from build123d import *

# Parameters (mm, degrees)
F1_DEPTH = 3
F2_DEPTH = 17
F3_R     = 5
F4_R     = 5
F5_R     = 2


with BuildPart() as f1:
    # F0 (on Top) → F1 (new body)
    with BuildSketch(Plane.XY):
        Polygon((-13.561376, 18.665632), (-57.446909, 18.665632), (-21.942767, -7.129637), (-35.504142, -48.867259), (0, -23.07199), (35.504142, -48.867259), (21.942767, -7.129637), (57.446909, 18.665632), (13.561376, 18.665632), (0, 60.403254), align=None)
        with BuildLine():
            Line((-37.903616, 13.665631), (-9.928662, 13.665631))
            Line((-9.928662, 13.665631), (-1.283926, 40.271394))
            ThreePointArc((-1.283926, 40.271394), (0, 41.204221), (1.283926, 40.271394))
            Line((1.283926, 40.271394), (9.928662, 13.665631))
            Line((9.928662, 13.665631), (37.903616, 13.665631))
            ThreePointArc((37.903616, 13.665631), (39.187542, 12.732804), (38.697126, 11.223459))
            Line((38.697126, 11.223459), (16.064913, -5.219807))
            Line((16.064913, -5.219807), (24.709649, -31.825569))
            ThreePointArc((24.709649, -31.825569), (24.219233, -33.334915), (22.632213, -33.334915))
            Line((22.632213, -33.334915), (0, -16.891649))
            Line((0, -16.891649), (-22.632213, -33.334915))
            ThreePointArc((-22.632213, -33.334915), (-24.219233, -33.334915), (-24.709649, -31.825569))
            Line((-24.709649, -31.825569), (-16.064913, -5.219807))
            Line((-16.064913, -5.219807), (-38.697126, 11.223459))
            ThreePointArc((-38.697126, 11.223459), (-39.187542, 12.732804), (-37.903616, 13.665631))
        make_face(mode=Mode.SUBTRACT)
        with BuildLine():
            Line((-1.283926, 40.271394), (-9.928662, 13.665631))
            Line((-9.928662, 13.665631), (-37.903616, 13.665631))
            ThreePointArc((-37.903616, 13.665631), (-39.187542, 12.732804), (-38.697126, 11.223459))
            Line((-38.697126, 11.223459), (-16.064913, -5.219807))
            Line((-16.064913, -5.219807), (-24.709649, -31.825569))
            ThreePointArc((-24.709649, -31.825569), (-24.219233, -33.334915), (-22.632213, -33.334915))
            Line((-22.632213, -33.334915), (0, -16.891649))
            Line((0, -16.891649), (22.632213, -33.334915))
            ThreePointArc((22.632213, -33.334915), (24.219233, -33.334915), (24.709649, -31.825569))
            Line((24.709649, -31.825569), (16.064913, -5.219807))
            Line((16.064913, -5.219807), (38.697126, 11.223459))
            ThreePointArc((38.697126, 11.223459), (39.187542, 12.732804), (37.903616, 13.665631))
            Line((37.903616, 13.665631), (9.928662, 13.665631))
            Line((9.928662, 13.665631), (1.283926, 40.271394))
            ThreePointArc((1.283926, 40.271394), (0, 41.204221), (-1.283926, 40.271394))
        make_face()
        with BuildLine():
            Line((-23.948804, -32.072782), (-15.124457, -4.914234))
            Line((-15.124457, -4.914234), (-38.226898, 11.870672))
            ThreePointArc((-38.226898, 11.870672), (-38.426697, 12.485591), (-37.903616, 12.865631))
            Line((-37.903616, 12.865631), (-9.347428, 12.865631))
            Line((-9.347428, 12.865631), (-0.523081, 40.02418))
            ThreePointArc((-0.523081, 40.02418), (0, 40.404221), (0.523081, 40.02418))
            Line((0.523081, 40.02418), (9.347428, 12.865631))
            Line((9.347428, 12.865631), (37.903616, 12.865631))
            ThreePointArc((37.903616, 12.865631), (38.426697, 12.485591), (38.226898, 11.870672))
            Line((38.226898, 11.870672), (15.124457, -4.914234))
            Line((15.124457, -4.914234), (23.948804, -32.072782))
            ThreePointArc((23.948804, -32.072782), (23.749005, -32.687701), (23.102441, -32.687701))
            Line((23.102441, -32.687701), (0, -15.902795))
            Line((0, -15.902795), (-23.102441, -32.687701))
            ThreePointArc((-23.102441, -32.687701), (-23.749005, -32.687701), (-23.948804, -32.072782))
        make_face(mode=Mode.SUBTRACT)
    extrude(amount=-F1_DEPTH)

    # F0 (on Top) → F2 (join)
    with BuildSketch(Plane.XY):
        with BuildLine():
            Line((-1.283926, 40.271394), (-9.928662, 13.665631))
            Line((-9.928662, 13.665631), (-37.903616, 13.665631))
            ThreePointArc((-37.903616, 13.665631), (-39.187542, 12.732804), (-38.697126, 11.223459))
            Line((-38.697126, 11.223459), (-16.064913, -5.219807))
            Line((-16.064913, -5.219807), (-24.709649, -31.825569))
            ThreePointArc((-24.709649, -31.825569), (-24.219233, -33.334915), (-22.632213, -33.334915))
            Line((-22.632213, -33.334915), (0, -16.891649))
            Line((0, -16.891649), (22.632213, -33.334915))
            ThreePointArc((22.632213, -33.334915), (24.219233, -33.334915), (24.709649, -31.825569))
            Line((24.709649, -31.825569), (16.064913, -5.219807))
            Line((16.064913, -5.219807), (38.697126, 11.223459))
            ThreePointArc((38.697126, 11.223459), (39.187542, 12.732804), (37.903616, 13.665631))
            Line((37.903616, 13.665631), (9.928662, 13.665631))
            Line((9.928662, 13.665631), (1.283926, 40.271394))
            ThreePointArc((1.283926, 40.271394), (0, 41.204221), (-1.283926, 40.271394))
        make_face()
        with BuildLine():
            Line((-23.948804, -32.072782), (-15.124457, -4.914234))
            Line((-15.124457, -4.914234), (-38.226898, 11.870672))
            ThreePointArc((-38.226898, 11.870672), (-38.426697, 12.485591), (-37.903616, 12.865631))
            Line((-37.903616, 12.865631), (-9.347428, 12.865631))
            Line((-9.347428, 12.865631), (-0.523081, 40.02418))
            ThreePointArc((-0.523081, 40.02418), (0, 40.404221), (0.523081, 40.02418))
            Line((0.523081, 40.02418), (9.347428, 12.865631))
            Line((9.347428, 12.865631), (37.903616, 12.865631))
            ThreePointArc((37.903616, 12.865631), (38.426697, 12.485591), (38.226898, 11.870672))
            Line((38.226898, 11.870672), (15.124457, -4.914234))
            Line((15.124457, -4.914234), (23.948804, -32.072782))
            ThreePointArc((23.948804, -32.072782), (23.749005, -32.687701), (23.102441, -32.687701))
            Line((23.102441, -32.687701), (0, -15.902795))
            Line((0, -15.902795), (-23.102441, -32.687701))
            ThreePointArc((-23.102441, -32.687701), (-23.749005, -32.687701), (-23.948804, -32.072782))
        make_face(mode=Mode.SUBTRACT)
    extrude(amount=F2_DEPTH)

    # F3
    f3_edges = [f1.edges().sort_by_distance(p)[0] for p in [
        (-35.504142, -48.867259, -1.5),
        (-57.446909, 18.665632, -1.5),
        (35.504142, -48.867259, -1.5),
        (0, 60.403254, -1.5),
        (57.446909, 18.665632, -1.5),
    ]]
    fillet(f3_edges, radius=F3_R)

    # F4
    f4_edges = [f1.edges().sort_by_distance(p)[0] for p in [
        (-21.942767, -7.129637, -1.5),
        (-13.561376, 18.665632, -1.5),
        (13.561376, 18.665632, -1.5),
        (21.942767, -7.129637, -1.5),
        (0, -23.07199, -1.5),
    ]]
    fillet(f4_edges, radius=F4_R)

    # F5
    f5_edges = [f1.edges().sort_by_distance(p)[0] for p in [
        (-9.347428, 12.865631, 7),
        (-9.928662, 13.665631, 8.5),
        (9.928662, 13.665631, 8.5),
        (9.347428, 12.865631, 7),
        (16.064913, -5.219807, 8.5),
        (15.124457, -4.914234, 7),
        (-15.124457, -4.914234, 7),
        (-16.064913, -5.219807, 8.5),
        (0, -15.902795, 7),
        (0, -16.891649, 8.5),
    ]]
    fillet(f5_edges, radius=F5_R)


solid = f1.part
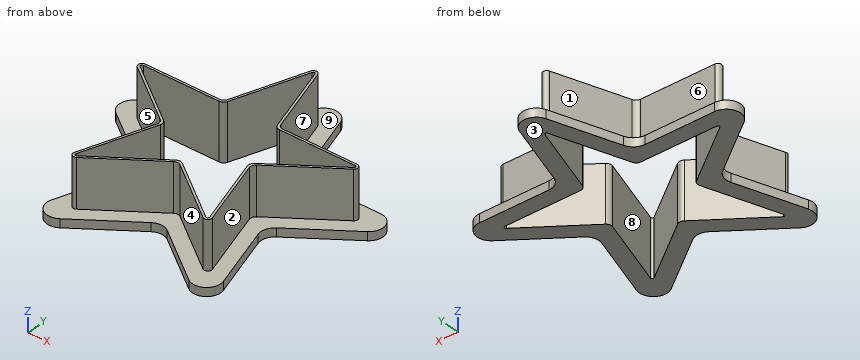
Could you check a few things on this model? Use its own coordinates, in mm. Face numbers are marked on the shaded views. A direction names the side the tool comes from. Round coordinates to 2 decimals unless told otherwise and drop trailing zeros. Order: outer loops, then holes, each group sorted by start corner. A loop starts at its lowest first (then second) coordinate and runs counter-clockwise, first axis right, second up.
(1) Which directions (+Z, -Z, +X, -X, +Y, -Y) give clear straight access to the entire face, cutting with the end or side of a thin tool? Please do the marked faces 5, 6, 7, 8 and 9.
Response values:
face 5: +Z, -X
face 6: +Z, -X, +Y
face 7: +Z, +X, +Y
face 8: +Z, -Z
face 9: +Z
(2) I'm going to push flat-ended pins straight in: pin 1 (8.5 mm diameter, centred on x = -20.5, z = 10.5, fed in from +Y); pin 2 (10 mm diameter, centred on y = 39.5, z = 9.5, fed in from +X); pin 3 (8 mm diameter, centred on y = -26, z = 10.5, fed in from -X). Where does each tip first touch, or does it pass through?
Response values:
pin 1: stops at y = 13.67
pin 2: stops at x = 3.16
pin 3: stops at x = -24.12
(3) Please list where these lines run through material, in increasing order: line 1 along X through (y, z) = (11.5, 14.75); line 2 along X through (y, z) = (-21, 4.25); line 3 along Y through (x, z) = (-32, 16.25).
Response values:
line 1: x = -38.98 to -37.72, 37.72 to 38.98
line 2: x = -21.19 to -20.35, -7.02 to -5.65, 5.65 to 7.02, 20.35 to 21.19
line 3: y = 6.36 to 7.35, 12.87 to 13.67
(4) Imagine slicing it at C-C (y = 17). Write out the boundary of the cut face in (x, z), plus the area to 3 significant figures.
Response values:
outline: (-45.78, -3) - (-8, -3) - (-8, 17) - (-8.85, 17) - (-8.85, 0) - (-45.78, 0) - close; (8, -3) - (45.78, -3) - (45.78, 0) - (8.85, 0) - (8.85, 17) - (8, 17) - close
area: 255 mm2
(5) Imagine slicing it at B-B (x = -29). Write out the boundary of the cut face in (y, z), plus the area to 3 significant figures.
Response values:
outline: (-39.77, -3) - (-28.85, -3) - (-28.85, 0) - (-39.77, 0) - close; (-2, -3) - (5.17, -3) - (5.17, 17) - (4.18, 17) - (4.18, 0) - (-2, 0) - close; (12.87, -3) - (18.67, -3) - (18.67, 0) - (13.67, 0) - (13.67, 17) - (12.87, 17) - close
area: 102 mm2
(6) Imagine slicing it at A-A (y = -20.5). Write out the boundary of the cut face in (x, z).
Response values:
outline: (-26.29, -3) - (-20.19, -3) - (-20.19, 17) - (-21.03, 17) - (-21.03, 0) - (-26.29, 0) - close; (-6.33, -3) - (6.33, -3) - (6.33, 17) - (4.97, 17) - (4.97, 0) - (-4.97, 0) - (-4.97, 17) - (-6.33, 17) - close; (20.19, -3) - (26.29, -3) - (26.29, 0) - (21.03, 0) - (21.03, 17) - (20.19, 17) - close
(7) Imagine slicing it at D-D (x = 35). Write out the boundary of the cut face in (y, z), plus the area to 3 significant figures.
Response values:
outline: (2.36, -3) - (9.53, -3) - (9.53, 17) - (8.54, 17) - (8.54, 0) - (2.36, 0) - close; (12.87, -3) - (18.67, -3) - (18.67, 0) - (13.67, 0) - (13.67, 17) - (12.87, 17) - close
area: 69.3 mm2
(8) If we mould it in two halves opening along X, with no side actions, what happens to the marked faces 1, 2, 3 and 4? For each: released by +X, released by -X, zero draft, split by the parting line, or undercut.
Response values:
face 1: released by -X
face 2: released by +X
face 3: zero draft
face 4: undercut
